```python
from build123d import *

# Parameters (mm, degrees)
F1_DEPTH = 63.5
F2_DEPTH = 50.8
F3_DEPTH = 15.875
F4_R     = 6.35


with BuildPart() as f1:
    # F0 (on Front) → F1 (new body, symmetric)
    with BuildSketch(Plane.XZ):
        Polygon((22.225, 18.464241), (-41.275, 18.464241), (-41.275, -18.464241), (41.275, -18.464241), (41.275, 18.464241), align=None)
    extrude(amount=F1_DEPTH, both=True)

    # F0 (on Front) → F2 (join)
    with BuildSketch(Plane.XZ):
        with BuildLine():
            add(Edge.make_bspline(
                [(-41.275, 18.464241), (-21.691592, 45.134176), (15.657064, 55.939447), (57.15, 53.389241)],
                knots=[0, 0, 0, 0, 104.437715, 104.437715, 104.437715, 104.437715], degree=3))
            Line((-41.275, 18.464241), (22.225, 18.464241))
            ThreePointArc((22.225, 18.464241), (32.454296, 43.159945), (57.15, 53.389241))
        make_face()
        Polygon((22.225, 18.464241), (-41.275, 18.464241), (-41.275, -18.464241), (41.275, -18.464241), (41.275, 18.464241), align=None)
        with BuildLine():
            ThreePointArc((57.15, 53.389241), (32.454296, 43.159945), (22.225, 18.464241))
            Line((22.225, 18.464241), (41.275, 18.464241))
            ThreePointArc((41.275, 18.464241), (45.92468, 29.689561), (57.15, 34.339241))
            Line((57.15, 34.339241), (69.494901, 34.339241))
            Line((69.494901, 34.339241), (69.494901, 53.000192))
            Line((69.494901, 53.000192), (69.494901, 53.389241))
            Line((69.494901, 53.389241), (57.15, 53.389241))
        make_face()
        Polygon((69.494901, 57.735759), (69.494901, 53.389241), (69.494901, 53.000192), (69.494901, 34.339241), (69.494901, 29.160759), (120.294901, 29.160759), (120.294901, 57.735759), align=None)
    extrude(amount=F2_DEPTH)

    # F0 (on Front) → F3 (join)
    with BuildSketch(Plane.XZ):
        with BuildLine():
            add(Edge.make_bspline(
                [(-41.275, 18.464241), (-21.691592, 45.134176), (15.657064, 55.939447), (57.15, 53.389241)],
                knots=[0, 0, 0, 0, 104.437715, 104.437715, 104.437715, 104.437715], degree=3))
            Line((-41.275, 18.464241), (22.225, 18.464241))
            ThreePointArc((22.225, 18.464241), (32.454296, 43.159945), (57.15, 53.389241))
        make_face()
        Polygon((22.225, 18.464241), (-41.275, 18.464241), (-41.275, -18.464241), (41.275, -18.464241), (41.275, 18.464241), align=None)
        with BuildLine():
            ThreePointArc((57.15, 53.389241), (32.454296, 43.159945), (22.225, 18.464241))
            Line((22.225, 18.464241), (41.275, 18.464241))
            ThreePointArc((41.275, 18.464241), (45.92468, 29.689561), (57.15, 34.339241))
            Line((57.15, 34.339241), (69.494901, 34.339241))
            Line((69.494901, 34.339241), (69.494901, 53.000192))
            Line((69.494901, 53.000192), (69.494901, 53.389241))
            Line((69.494901, 53.389241), (57.15, 53.389241))
        make_face()
        Polygon((69.494901, 57.735759), (69.494901, 53.389241), (69.494901, 53.000192), (69.494901, 34.339241), (69.494901, 29.160759), (120.294901, 29.160759), (120.294901, 57.735759), align=None)
    extrude(amount=F3_DEPTH)

    # F4
    f4_edges = [f1.edges().sort_by_distance(p)[0] for p in [
        (41.275, -63.5, 0),
        (-41.275, -63.5, 0),
        (41.275, 63.5, 0),
        (-41.275, 63.5, 0),
    ]]
    fillet(f4_edges, radius=F4_R)


solid = f1.part
```
Here's how the part is built. I have some questions about the finished solid (model axes, mm). A direction names the side the tool comes from. Give positions to 0.01 mm unless a question says otherwise; leave off trailing zeros. Loops run counter-clockwise (first coordinate to the right, second up) from the corner with the lowest first, then second, coordinate; pieces in that order, holes last. Notation, with made-up numbers: M 9.25,-38.5 L 20.25,-38.5 A24 cw 20.25,-16.5 Z; hole C 56.5,-10.5 d1. An arc over 180 degrees is marked long. Return JSON: item names as keys, results as strings.
Item 1: Please list where these lines run through material, in increasing order: line 1 (Y direction, x = 30, z = 50); line 2 (X direction, y = -41, z = 13.5) (3 decimals); line 3 (Z direction, x = 100, y = -20.5).
A:
{"line 1": "y = -50.8 to 0", "line 2": "x = -41.275 to 41.275", "line 3": "z = 29.16 to 57.74"}
Item 2: Imagine slicing it at B-B on y = 30. List the corners of the cut face in (x, z) for me (3 decimals).
A:
{"outline": "M -41.275,-18.464 L 41.275,-18.464 L 41.275,18.464 L -41.275,18.464 Z"}
Item 3: Imagine slicing it at C-C on x = 94.5. List the corners of the cut face in (y, z) for me, then the cut area to 3 significant figures.
A:
{"outline": "M -50.8,29.16 L 0,29.16 L 0,57.74 L -50.8,57.74 Z", "area": "1,450 mm^2"}
Item 4: On a 3-axis mill with a long thin cutter (end or side, diameter ignored), from which of +Z, -Z, +X, -X, +Y, -Y can I reach the whole of each face in a straight line? I mean faces 1 (the cylindrical face through (45.802, -25.044, 29.565)), 2 (the flat face through (41.275, 1, 0)), 3 (the flat face through (1, 31, 18.464)). Say none if no direction works.
A:
{"face 1": "-Z, +Y, -Y", "face 2": "-Z, +X, +Y, -Y", "face 3": "+Z, +X, -X, +Y"}
Item 5: I'm going to push flat-ended pins straight in: pin 1 Ø18.5 at (y, z) = (14.5, -1) entering from +X (3 decimals); pin 2 Ø13.5 at (x, y) = (63.5, -19) entering from -Z; pin 3 Ø10 at (x, z) = (27, 22.5) entering from +Y; pin 4 Ø1.5 at (x, z) = (85.5, 27.5) entering from -Y. Where does each tip first touch, or does it pass through?
A:
{"pin 1": "stops at x = 41.275", "pin 2": "stops at z = 29.16", "pin 3": "stops at y = 63.5", "pin 4": "passes through"}
Item 6: Thinking about a two-plate mould opening in X: for faces 4 (the cylindrical face through (-39.365, -61.689, -0.258)), 5 (the flat face through (0, 63.5, 0)), 6 (the flat face through (63, -25, 34.339)), which applies, released by +X, released by -X, zero draft, split by the parting line, or undercut?
A:
{"face 4": "released by -X", "face 5": "zero draft", "face 6": "undercut"}
Item 7: Imagine slicing it at A-A on z = 10.5. List the corners of the cut face in (x, y) for me (3 decimals).
A:
{"outline": "M -41.275,-57.15 A6.35 ccw -34.925,-63.5 L 34.925,-63.5 A6.35 ccw 41.275,-57.15 L 41.275,57.15 A6.35 ccw 34.925,63.5 L -34.925,63.5 A6.35 ccw -41.275,57.15 Z"}
